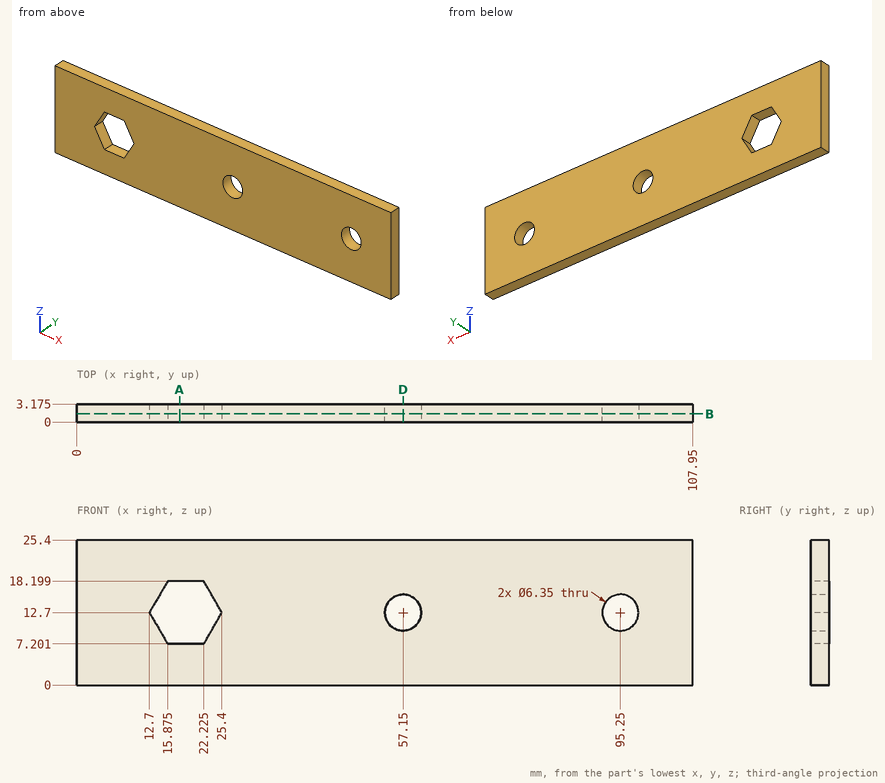
Input: dimensioned drawing with shaded views. Units: mm. Origin: part minimum x, y, z. Give positions to 0.01 mm unless a question says otherwise; leave off trailing zeros. Order: outer loops, then holes, each group sorted by start corner. A loop starts at its lowest first (then second) coordinate and runs counter-clockwise, first axis right, second up.
(1) Section query B-B (y = 1.45). State how many separate pieces and enclosed holes the cut face has, plus the area to 3 significant figures.
(2) Section query D-D (x = 57.15). Return the cut outline in (y, z) (1 decimal).
(3) Material intervals for line 1 along Z through (x, y) = (95.25, 0.75) (1 decimal); line 2 along Z through (x, y) = (19, 0.8); line 3 along X through (y, z) = (1.3, 8.75), sorted ascending.
(4) Section query A-A (x = 18). Return the cut outline in (y, z) (1 decimal).
(5) Contact query for a flat-ended pin moving along its axis: P1, Ø5, axis at x = 95.25, z = 12.7, coming from the -Y side. Output: stop coordinate, or through.
Outcome:
1. separate pieces: 1
1. enclosed holes: 3
1. area: 2,570 mm2
2. outline: (0, 0) - (3.2, 0) - (3.2, 9.5) - (0, 9.5) - close; (0, 15.9) - (3.2, 15.9) - (3.2, 25.4) - (0, 25.4) - close
3. line 1: z = 0 to 9.5, 15.9 to 25.4
3. line 2: z = 0 to 7.2, 18.2 to 25.4
3. line 3: x = 0 to 14.98, 23.12 to 107.95
4. outline: (0, 0) - (3.2, 0) - (3.2, 7.2) - (0, 7.2) - close; (0, 18.2) - (3.2, 18.2) - (3.2, 25.4) - (0, 25.4) - close
5. P1: passes through
